```python
from build123d import *

# Parameters (mm, degrees)
SKETCH028_R     = 3.8
PAD007_DEPTH    = 10
CHAMFER003_SIZE = 1
FILLET008_R     = 1


with BuildPart() as part:
    # Sketch028 → Pad007 (new body)
    with BuildSketch(Plane.XY):
        Circle(SKETCH028_R)
    extrude(amount=PAD007_DEPTH)

    # Sketch029 → Groove002 (revolve, cut)
    with BuildSketch(Plane.XZ):
        with BuildLine():
            Line((-2.3, 10), (0, 10))
            Line((0, 1.6), (0, 10))
            Line((0, 1.6), (-2.3, 1.6))
            ThreePointArc((-2.3, 1.6), (-1.741466, 2.552438), (-1.85, 3.651219))
            ThreePointArc((-1.85, 5.08374), (-2, 4.367479), (-1.85, 3.651219))
            ThreePointArc((-1.85, 5.08374), (-1.7, 5.8), (-1.85, 6.51626))
            ThreePointArc((-1.85, 7.948781), (-2, 7.232521), (-1.85, 6.51626))
            ThreePointArc((-1.85, 7.948781), (-1.741466, 9.047562), (-2.3, 10))
        make_face()
    revolve(axis=Axis((0, 0, 0), (0, 0, 1)), mode=Mode.SUBTRACT)

    # Chamfer003
    chamfer003_edges = [part.edges().sort_by_distance(p)[0] for p in [
        (-3.8, 0, 0),
    ]]
    chamfer(chamfer003_edges, length=CHAMFER003_SIZE)

    # Fillet008
    fillet008_edges = [part.edges().sort_by_distance(p)[0] for p in [
        (-3.8, 0, 1),
    ]]
    fillet(fillet008_edges, radius=FILLET008_R)


solid = part.part
```
Check sheet for the modelled part. Datum: model origin and axes. Units: mm. Give positions to 0.01 mm unless a question says otherwise; leave off trailing zeros. Write each loop counter-clockwise with the first axis right and the second up, starting at its lowest first coordinate (ties: lowest second). Pieces come first, ordered by that corner, then holes.
Item 1: Gauge pin test, flat end, axial feed: pin 1 (4 mm diameter, centred on x = -2, y = -1, fed in from +Z). Record the tip position at first contact, or that the pin passes through.
Item 2: Cross-section at B-B (z = 9.25). Enter the section's corners in (x, y).
Item 3: Draft check along Y on faces 1 (the face through (2, -2, 10)), 2 (the face through (0, 0, 1.6)), 3 (the face through (-3.796, 0.167, 5.647)). Enter one of: released by +Y, released by -Y, zero draft, split by the parting line, or undercut.
Item 4: Scan lines: L1, parallel to Y at x = -1.5, z = 5.5; L2, parallel to Y at x = -0.75, z = 7.5; L3, parallel to X at y = -1, z = 8.5. Record each from-to range of solid material in increasing order.
Item 5: Cross-section at A-A (z = 2.25). Enter the section's corners in (x, y), and give its area (3 significant figures).
Report:
1. pin 1: stops at z = 10
2. outline: circle Ø7.6 at (0, 0); hole circle Ø3.6 at (0, 0)
3. face 1: zero draft
3. face 2: undercut
3. face 3: split by the parting line
4. L1: y = -3.49 to -0.85, 0.85 to 3.49
4. L2: y = -3.73 to -1.83, 1.83 to 3.73
4. L3: x = -3.67 to -1.38, 1.38 to 3.67
5. outline: circle Ø7.6 at (0, 0); hole circle Ø3.67 at (0, 0)
5. area: 34.8 mm2
